```python
from build123d import *

# Parameters (mm, degrees)
F1_DEPTH = 34.3916
F2_START = 31.8516
F0_W     = 5.08
F0_H     = 2.54
F2_DEPTH = 5.08
F3_START = -31.8516
F3_DEPTH = 5.08


with BuildPart() as f1:
    # F0 (on Right) → F1 (new body, symmetric)
    with BuildSketch(Plane.YZ):
        with BuildLine():
            Line((82.1398573303, 169.3418), (79.5998573303, 169.3418))
            Line((79.5998573303, 169.3418), (79.5998573303, 164.5491375))
            ThreePointArc((79.5998573303, 164.5491375), (80.3438061061, 162.7530862758), (82.1398573303, 162.0091375))
            Line((82.1398573303, 162.0091375), (100.203, 162.0091375))
            Line((100.203, 162.0091375), (100.203, 164.5491375))
            Line((100.203, 164.5491375), (89.6502663064, 164.5491375))
            Line((89.6502663064, 164.5491375), (84.5702663064, 164.5491375))
            Line((84.5702663064, 164.5491375), (82.1398573303, 164.5491375))
            Line((82.1398573303, 164.5491375), (82.1398573303, 169.3418))
        make_face()
        with BuildLine():
            Line((120.8061426697, 169.3418), (118.2661426697, 169.3418))
            Line((118.2661426697, 169.3418), (118.2661426697, 164.5491375))
            Line((118.2661426697, 164.5491375), (115.8357336936, 164.5491375))
            Line((115.8357336936, 164.5491375), (110.7557336936, 164.5491375))
            Line((110.7557336936, 164.5491375), (100.203, 164.5491375))
            Line((100.203, 164.5491375), (100.203, 162.0091375))
            Line((100.203, 162.0091375), (118.2661426697, 162.0091375))
            ThreePointArc((118.2661426697, 162.0091375), (120.0621938939, 162.7530862758), (120.8061426697, 164.5491375))
            Line((120.8061426697, 164.5491375), (120.8061426697, 169.3418))
        make_face()
    extrude(amount=F1_DEPTH, both=True)

    # F0 (on Right) → F2 (join)
    with BuildSketch(Plane.YZ.offset(F2_START)):
        with Locations((87.1102663064, 165.8191375)):
            Rectangle(F0_W, F0_H)
        with Locations((113.2957336936, 165.8191375)):
            Rectangle(F0_W, F0_H)
    extrude(amount=F2_DEPTH)

    # F0 (on Right) → F3 (join)
    with BuildSketch(Plane.YZ.offset(F3_START)):
        with Locations((87.1102663064, 165.8191375)):
            Rectangle(F0_W, F0_H)
        with Locations((113.2957336936, 165.8191375)):
            Rectangle(F0_W, F0_H)
    extrude(amount=-F3_DEPTH)


solid = f1.part
```
Can you work these out from the model? Positions are in its coordinate system, mm. A direction names the side the tool comes from. Give positions to 0.01 mm unless a question says otherwise; leave off trailing zeros. Write each loop counter-clockwise with the first axis right and the second up, starting at its lowest first coordinate (ties: lowest second). Pieces come first, ordered by that corner, then holes. Notation, with made-up numbers: (83, 20.5) - (108, 20.5) arc R31 cw to (108, 55.5) - close; hole circle Ø6 at (21.25, 74). An arc over 180 degrees is marked (long way). Write item = value, one per line. Start each with the question number.
1. On a 3-axis mill with a long thin cutter (end or side, diameter ignored), from which of +Z, -Z, +X, -X, +Y, -Y can I reach the whole of each face in a straight line? I mean faces 1 (the face through (34, 115.836, 166)), 2 (the face through (31.852, 87, 166)), 3 (the face through (36.932, 87, 166)). Say none if no direction works.
2. Please list where these lines run through material, in increasing order: line 1 (X direction, y = 113.5, z = 165.5); line 2 (Y direction, x = 33, z = 167.75); line 3 (Z direction, x = -30, y = 115).
3. For pin 1 (2 mm diameter, centred on x = -35.5, z = 166, fed in from -Y); pin 2 (1.5 mm diameter, centred on x = 1.5, y = 87, fed in from +Z); pin 3 (1.5 mm diameter, centred on x = -33.5, y = 87, fed in from +Z), each with a flat end and sliding along its axis, tell me the tip position at first contact or that it passes through.
4. Imagine slicing it at C-C (y = 86.5). Please give me the cut outline in (x, z).
5. Imagine slicing it at A-A (z = 168). Please give me the cut outline in (x, y), and give its area (3 significant figures).
6. Thinking about a two-plate mould opening in Y: for faces 4 (the face through (-36, 113, 164.549)), 5 (the face through (0, 120.806, 167)), 6 (the face through (0, 118.266, 167)), which applies, released by +Y, released by -Y, zero draft, split by the parting line, or undercut?
7. Imagine slicing it at B-B (x = -17.5). Please give me the cut outline in (y, z).
8. Imagine slicing it at D-D (z = 163.5). Please give me the cut outline in (x, y), and give its area (3 significant figures).
Worked answers:
q1.face_1 = +Z, +X, -X
q1.face_2 = +Z
q1.face_3 = +Z, -Z, +X, +Y, -Y
q2.line_1 = -36.93 to -31.85, 31.85 to 36.93
q2.line_2 = 79.6 to 82.14, 118.27 to 120.81
q2.line_3 = 162.01 to 164.55
q3.pin_1 = 84.57
q3.pin_2 = 164.55
q3.pin_3 = 167.09
q4.outline = (-36.93, 164.55) - (-34.39, 164.55) - (-34.39, 162.01) - (34.39, 162.01) - (34.39, 164.55) - (36.93, 164.55) - (36.93, 167.09) - (31.85, 167.09) - (31.85, 164.55) - (-31.85, 164.55) - (-31.85, 167.09) - (-36.93, 167.09) - close
q5.outline = (-34.39, 79.6) - (34.39, 79.6) - (34.39, 82.14) - (-34.39, 82.14) - close; (-34.39, 118.27) - (34.39, 118.27) - (34.39, 120.81) - (-34.39, 120.81) - close
q5.area = 349 mm2
q6.face_4 = zero draft
q6.face_5 = released by +Y
q6.face_6 = undercut
q7.outline = (79.6, 164.55) arc R2.54 ccw to (82.14, 162.01) - (118.27, 162.01) arc R2.54 ccw to (120.81, 164.55) - (120.81, 169.34) - (118.27, 169.34) - (118.27, 164.55) - (82.14, 164.55) - (82.14, 169.34) - (79.6, 169.34) - close
q8.outline = (-34.39, 79.83) - (34.39, 79.83) - (34.39, 120.58) - (-34.39, 120.58) - close
q8.area = 2,800 mm2
